from build123d import *

# Parameters (mm, degrees)
SKETCH1_R            = 8.525
BOSS_EXTRUDE11_DEPTH = 4
SKETCH20_R           = 8.575
BOSS_EXTRUDE12_DEPTH = 4
SKETCH21_R           = 9.5
BOSS_EXTRUDE13_DEPTH = 1.25
SKETCH22_R           = 8.55
BOSS_EXTRUDE14_DEPTH = 7
SKETCH30_R           = 8.525
BOSS_EXTRUDE15_DEPTH = 15
SKETCH33_R           = 2.1
CUT_EXTRUDE14_DEPTH  = 5.8
BOSS_EXTRUDE16_START = 1.5
SKETCH35_R           = 9.5
BOSS_EXTRUDE16_DEPTH = 1.5
SKETCH36_R           = 1.6
CUT_EXTRUDE15_DEPTH  = 31.25
CIRPATTERN1_COUNT    = 2
SKETCH43_R           = 1.55
CUT_EXTRUDE20_DEPTH  = 31.25
SKETCH44_R           = 2
CUT_EXTRUDE21_DEPTH  = 4
CUT_EXTRUDE22_DEPTH  = 3
CUT_EXTRUDE23_DEPTH  = 3
SKETCH47_W           = 22.343806143
SKETCH47_H           = 21.789827479
CUT_EXTRUDE24_DEPTH  = 12.25
SKETCH48_W           = 6
SKETCH48_H           = 6
CUT_EXTRUDE25_DEPTH  = 3


with BuildPart() as part:
    # Sketch1 → Boss-Extrude11 (new body)
    with BuildSketch(Plane(origin=(0, 0, 0), x_dir=(1, 0, 0), z_dir=(0, 1, 0))):
        with Locations(Location((0, 0, 0), (0, 0, 270))):
            Circle(SKETCH1_R)
    extrude(amount=BOSS_EXTRUDE11_DEPTH)

    # Sketch20 → Boss-Extrude12 (add)
    with BuildSketch(Plane(origin=(0, 4, 0), x_dir=(1, 0, 0), z_dir=(0, 1, 0))):
        with Locations(Location((1.2, 0, 0), (0, 0, 96.402715722))):
            Circle(SKETCH20_R)
    extrude(amount=BOSS_EXTRUDE12_DEPTH)

    # Sketch21 → Boss-Extrude13 (add)
    with BuildSketch(Plane(origin=(0, 8, 0), x_dir=(1, 0, 0), z_dir=(0, 1, 0))):
        with Locations(Location((0.6, 0, 0), (0, 0, 270))):
            Circle(SKETCH21_R)
    extrude(amount=BOSS_EXTRUDE13_DEPTH)

    # Sketch22 → Boss-Extrude14 (add)
    with BuildSketch(Plane(origin=(0, 9.25, 0), x_dir=(1, 0, 0), z_dir=(0, 1, 0))):
        with Locations(Location((0.6, 0, 0), (0, 0, 270))):
            Circle(SKETCH22_R)
    extrude(amount=BOSS_EXTRUDE14_DEPTH)

    # Sketch30 → Boss-Extrude15 (add)
    with BuildSketch(Plane.XZ):
        with Locations(Location((0.6, 0, 0), (0, 0, 92.01669015))):
            Circle(SKETCH30_R)
    extrude(amount=BOSS_EXTRUDE15_DEPTH)

    # Sketch33 → Cut-Extrude14 (cut)
    with BuildSketch(Plane.XZ.offset(15)):
        with Locations(Location((0.6, 0, 0), (0, 0, 270))):
            Circle(SKETCH33_R)
    extrude(amount=-CUT_EXTRUDE14_DEPTH, mode=Mode.SUBTRACT)

    # Sketch35 → Boss-Extrude16 (add)
    with BuildSketch(Plane.XZ.offset(BOSS_EXTRUDE16_START)):
        with Locations(Location((0.6, 0, 0), (0, 0, 90))):
            Circle(SKETCH35_R)
    extrude(amount=-BOSS_EXTRUDE16_DEPTH)

    # Sketch36 → Cut-Extrude15 (cut)
    with BuildSketch(Plane.XZ.offset(15)):
        with Locations(Location((0.6, 6, 0), (0, 0, 270))):
            Circle(SKETCH36_R)
    cut_extrude15 = extrude(amount=-CUT_EXTRUDE15_DEPTH, mode=Mode.SUBTRACT)

    # CirPattern1: Cut-Extrude15 ×2 about axis
    cirpattern1_axis = Axis((0.6, 0, 0), (0, 1, 0))
    for i in range(1, CIRPATTERN1_COUNT):
        add(cut_extrude15.rotate(cirpattern1_axis, i * 360 / CIRPATTERN1_COUNT), mode=Mode.SUBTRACT)

    # Sketch43 → Cut-Extrude20 (cut)
    with BuildSketch(Plane.XZ.offset(15)):
        with Locations(Location((-4.9, 0, 0), (0, 0, 270))):
            Circle(SKETCH43_R)
        with Locations(Location((6.1, 0, 0), (0, 0, 270))):
            Circle(SKETCH43_R)
    extrude(amount=-CUT_EXTRUDE20_DEPTH, mode=Mode.SUBTRACT)

    # Sketch44 → Cut-Extrude21 (cut)
    with BuildSketch(Plane(origin=(0, 16.25, 0), x_dir=(1, 0, 0), z_dir=(0, 1, 0))):
        with Locations(Location((-4.9, 0, 0), (0, 0, 270))):
            Circle(SKETCH44_R)
        with Locations(Location((6.1, 0, 0), (0, 0, 270))):
            Circle(SKETCH44_R)
    extrude(amount=-CUT_EXTRUDE21_DEPTH, mode=Mode.SUBTRACT)

    # Sketch45 → Cut-Extrude22 (cut)
    with BuildSketch(Plane(origin=(0, 16.25, 0), x_dir=(1, 0, 0), z_dir=(0, 1, 0))):
        with BuildLine():
            Line((-2.4, -6), (-2.4, -10.872564071))
            Line((-2.4, -10.872564071), (3.6, -10.872564071))
            Line((3.6, -10.872564071), (3.6, -6))
            ThreePointArc((3.6, -6), (0.6, -3), (-2.4, -6))
        make_face()
        with BuildLine():
            Line((-2.4, 6), (-2.4, 11.42214608))
            Line((-2.4, 11.42214608), (3.6, 11.42214608))
            Line((3.6, 11.42214608), (3.6, 6))
            ThreePointArc((3.6, 6), (0.6, 3), (-2.4, 6))
        make_face()
    extrude(amount=-CUT_EXTRUDE22_DEPTH, mode=Mode.SUBTRACT)

    # Sketch46 → Cut-Extrude23 (cut)
    with BuildSketch(Plane.XZ.offset(15)):
        with BuildLine():
            Line((-4.9, 3), (-9.719928829, 3))
            Line((-9.719928829, 3), (-9.719928829, -3))
            Line((-9.719928829, -3), (-4.9, -3))
            ThreePointArc((-4.9, -3), (-1.9, 0), (-4.9, 3))
        make_face()
        with BuildLine():
            Line((6.1, 3), (10.889396495, 3))
            Line((10.889396495, 3), (10.889396495, -3))
            Line((10.889396495, -3), (6.1, -3))
            ThreePointArc((6.1, -3), (3.1, 0), (6.1, 3))
        make_face()
    extrude(amount=-CUT_EXTRUDE23_DEPTH, mode=Mode.SUBTRACT)

    # Sketch47 → Cut-Extrude24 (cut)
    with BuildSketch(Plane(origin=(0, 16.25, 0), x_dir=(1, 0, 0), z_dir=(0, 1, 0))):
        with Locations((0.37577054, -0.013189968)):
            Rectangle(SKETCH47_W, SKETCH47_H)
    extrude(amount=-CUT_EXTRUDE24_DEPTH, mode=Mode.SUBTRACT)

    # Sketch48 → Cut-Extrude25 (cut)
    with BuildSketch(Plane(origin=(0, 4, 0), x_dir=(1, 0, 0), z_dir=(0, 1, 0))):
        with Locations((0.6, 0)):
            Rectangle(SKETCH48_W, SKETCH48_H)
    extrude(amount=-CUT_EXTRUDE25_DEPTH, mode=Mode.SUBTRACT)


solid = part.part
Verification items for the finished model (mm, model axes). A direction names the side the tool comes from. Coordinates: 2 decimals unless noted, no trailing zeros. Write each loop counter-clockwise with the first axis right and the second up, starting at its lowest first coordinate (ties: lowest second). Pieces come first, ordered by that corner, then holes. Notation, with made-up numbers: (-2, 60) -> (3, 60) arc R15 ccw to (3, 89) -> close; hole circle Ø7 at (-5, 22.25). An arc over 180 degrees is marked (long way). One line per item, written item: value. Start each with the question number.
Q1. Cross-section at A-A on z = 0. State how many separate pieces and enclosed holes the cut face has, and give its area (3 significant figures).
Q2. Cross-section at C-C on z = -6. Enter the section's corners in (x, y).
Q3. Mould release check, pull along X, two halves, no side actions. Record for faces 1 (the cylindrical face through (0.119, -5.633, -4.474)), 2 (the flat face through (7, -14, 3)), 3 (the cylindrical face through (-2.245, -8.156, 8.036)): pulls with the +X half, pulls with the -X half, needs draft (parallel to the pull), parting line crosses it, or undercut.
Q4. Go/stop test with flat-tipped pins: P1, Ø4, axis at x = 6.1, z = 0, coming from the -Y side; P2, Ø10, axis at x = 7, y = -5.5, coming from the +Z side; P3, Ø2, axis at x = 8, y = -14, coming from the +Z side. Record where each tip stops, or that it passes through.
Q5. Cross-section at B-B on x = 0. Enter the section's corners in (y, z) (3 decimals), and give its area (3 significant figures).
Q6. Cross-section at D-D on y = 2.75. Enter the section's corners in (x, z) (3 decimals), and give its area (3 significant figures).
Q7. Access from +Z, -Z, +X, -X, +Y, -Y to the whole of each face (thin tool, end or side, straight path). Record for faces 4 (the flat face through (-6, -14, -3)), 5 (the flat face through (3.6, 3, 0)), 6 (the flat face through (-3, -1.5, -8)), 7 (the cylindrical face through (9.874, -0.76, -2.059)), 8 (the flat face through (7.5, -12, 1.4)).
Q8. Thickness scan on L1, parallel to X at y = -4.25, z = 0 (3 decimals); L2, parallel to Z at x = -0.75, y = 2.25; L3, parallel to X at y = -10.7, z = 0 (3 decimals). Record the ranges inside material, lowest first. Write a range as from..to.
Checked values:
1. separate pieces: 3
1. enclosed holes: 0
1. area: 149 mm²
2. outline: (-6.77, -1.5) -> (-5.46, -1.5) -> (-5.46, -15) -> (-1, -15) -> (-1, 4) -> (-6.06, 4) -> (-6.06, 0) -> (-6.77, 0) -> close; (2.2, -15) -> (6.66, -15) -> (6.66, -1.5) -> (7.97, -1.5) -> (7.97, 0) -> (6.06, 0) -> (6.06, 4) -> (2.2, 4) -> close
3. face 1: undercut
3. face 2: needs draft
3. face 3: parting line crosses it
4. P1: stops at y = -12
4. P2: stops at z = 8.87
4. P3: stops at z = 5.63
5. outline: (-15, -8.504) -> (-1.5, -8.504) -> (-1.5, -9.481) -> (0, -9.481) -> (0, -8.525) -> (4, -8.525) -> (4, -7.483) -> (-15, -7.483) -> close; (-15, -4.517) -> (4, -4.517) -> (4, -3) -> (1, -3) -> (1, 3) -> (4, 3) -> (4, 4.517) -> (-15, 4.517) -> (-15, 2.012) -> (-9.2, 2.012) -> (-9.2, -2.012) -> (-15, -2.012) -> close; (-15, 7.483) -> (4, 7.483) -> (4, 8.525) -> (0, 8.525) -> (0, 9.481) -> (-1.5, 9.481) -> (-1.5, 8.504) -> (-15, 8.504) -> close
5. area: 172 mm²
6. outline: circle Ø17.05 at (0, 0); hole circle Ø3.1 at (-4.9, 0); hole (-2.4, -3) -> (3.6, -3) -> (3.6, 3) -> (-2.4, 3) -> close; hole circle Ø3.2 at (0.6, -6); hole circle Ø3.2 at (0.6, 6); hole circle Ø3.1 at (6.1, 0)
6. area: 161 mm²
7. face 4: -X, -Y
7. face 5: +Y
7. face 6: -Y
7. face 7: +Y, -Y
7. face 8: +X, -Y
8. L1: x = -7.925..-6.45, -3.35..4.55, 7.65..9.125
8. L2: z = -8.49..-6.86, -5.14..-3, 3..5.14, 6.86..8.49
8. L3: x = -7.925..-6.45, -3.35..-1.5, 2.7..4.55, 7.65..9.125
